```python
from build123d import *

# Parameters (mm, degrees)
F0_W     = 7.25
F0_H     = 3.25
F1_DEPTH = 3


with BuildPart() as f1:
    # F0 (on Top) → F1 (new body)
    with BuildSketch(Plane.XY):
        Polygon((9.582664, 28.182806), (4.046888, 28.182806), (-1.488889, 28.182806), (-11.920412, 38.29651), (-20.548956, 38.811646), (-21.450445, 36.493532), (-36.131848, 37.266236), (-36.775768, 39.455567), (-45.790665, 40.228274), (-51.328391, 34.561768), (-51.714741, 26.577145), (-47.207296, 25.546871), (-45.919452, 27.607419), (-31.366833, 24.001461), (-31.238047, 21.554559), (-26.953112, 20.524286), (-26.953112, 11.682806), (-26.953112, 2.841327), (-31.238047, 1.811053), (-31.366833, -0.635848), (-45.919452, -4.241806), (-47.207296, -2.181258), (-51.714741, -3.211532), (-51.328391, -11.196155), (-45.790665, -16.862661), (-36.775768, -16.089954), (-36.131848, -13.900623), (-21.450445, -13.127919), (-20.548956, -15.446034), (-11.920412, -14.930897), (-1.488889, -4.817194), (4.046888, -4.817194), (9.582664, -4.817194), (20.014187, -14.930897), (28.642732, -15.446034), (29.54422, -13.127919), (44.225623, -13.900623), (44.869543, -16.089954), (53.88444, -16.862661), (59.422166, -11.196155), (59.808516, -3.211532), (55.301071, -2.181258), (54.013227, -4.241806), (39.460608, -0.635848), (39.331823, 1.811053), (35.046888, 2.841327), (35.046888, 20.524286), (39.331823, 21.554559), (39.460608, 24.001461), (54.013227, 27.607419), (55.301071, 25.546871), (59.808516, 26.577145), (59.422166, 34.561768), (53.88444, 40.228274), (44.869543, 39.455567), (44.225623, 37.266236), (29.54422, 36.493532), (28.642732, 38.811646), (20.014187, 38.29651), align=None)
        Polygon((-47.588665, -8.516893), (-28.300909, -4.230727), (-26.597083, -9.545867), (-39.028991, -10.319404), (-39.857782, -12.695283), (-44.388525, -12.86104), (-47.648445, -9.766877), align=None, mode=Mode.SUBTRACT)
        with Locations((-11.828112, -3.192194)):
            Rectangle(F0_W, F0_H, mode=Mode.SUBTRACT)
        with Locations((19.921888, -3.192194)):
            Rectangle(F0_W, F0_H, mode=Mode.SUBTRACT)
        Polygon((34.690858, -9.545867), (36.394685, -4.230727), (55.68244, -8.516893), (55.74222, -9.766877), (52.482301, -12.86104), (47.951558, -12.695283), (47.122766, -10.319404), align=None, mode=Mode.SUBTRACT)
        Polygon((-9.203112, 9.764191), (-9.203112, 11.682806), (-9.203112, 13.601422), (-5.139121, 14.579791), (-5.063862, 15.55816), (-3.483421, 16.31075), (-2.580312, 15.934454), (0.806347, 17.364377), (0.430051, 18.192228), (2.010493, 18.944819), (4.046888, 18.944819), (6.083283, 18.944819), (7.663724, 18.192228), (7.287428, 17.364377), (10.674088, 15.934454), (11.577197, 16.31075), (13.157638, 15.55816), (13.232897, 14.579791), (17.296888, 13.601422), (17.296888, 11.682806), (17.296888, 9.764191), (13.232897, 8.785822), (13.157638, 7.807453), (11.577197, 7.054863), (10.674088, 7.431159), (7.287428, 6.001236), (7.663724, 5.173385), (6.083283, 4.420794), (4.046888, 4.420794), (2.010493, 4.420794), (0.430051, 5.173385), (0.806347, 6.001236), (-2.580312, 7.431159), (-3.483421, 7.054863), (-5.063862, 7.807453), (-5.139121, 8.785822), align=None, mode=Mode.SUBTRACT)
        Polygon((-26.597083, 32.911479), (-28.300909, 27.59634), (-47.588665, 31.882506), (-47.648445, 33.13249), (-44.388525, 36.226653), (-39.857782, 36.060896), (-39.028991, 33.685017), align=None, mode=Mode.SUBTRACT)
        with Locations((-11.828112, 26.557806)):
            Rectangle(F0_W, F0_H, mode=Mode.SUBTRACT)
        with Locations((19.921888, 26.557806)):
            Rectangle(F0_W, F0_H, mode=Mode.SUBTRACT)
        Polygon((36.394685, 27.59634), (34.690858, 32.911479), (47.122766, 33.685017), (47.951558, 36.060896), (52.482301, 36.226653), (55.74222, 33.13249), (55.68244, 31.882506), align=None, mode=Mode.SUBTRACT)
    extrude(amount=F1_DEPTH)


solid = f1.part
```
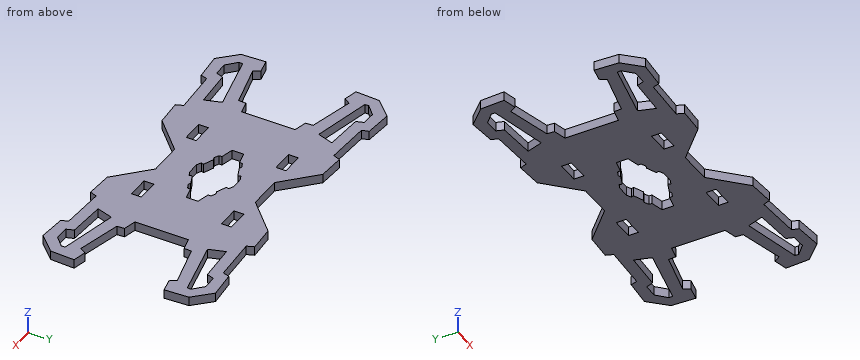
Here's how the part is built. I have some questions about the finished solid (model axes, mm). Coordinates: 2 decimals unless noted, no trailing zeros. Loops run counter-clockwise (first coordinate to the right, second up) from the corner with the lowest first, then second, coordinate; pieces in that order, holes last. Notation, with made-up numbers: M -2.5,-10.75 L 40.5,-10.75 A6 ccw 40.5,-2.75 Z; hole C -40,-20.5 d1. An arc over 180 degrees is marked long. One line per item, written item: value.
1. Imagine slicing it at A-A (y = 11.5). List the corners of the cut face in (x, z) for me, and give its area (4 significant figures).
Geometry says:
outline: M -26.95,0 L -9.2,0 L -9.2,3 L -26.95,3 Z; M 17.3,0 L 35.05,0 L 35.05,3 L 17.3,3 Z
area: 106.5 mm2
2. Will these pins go through, and if not, where does the flat tip stop? pin 1 Ø4 at (x, y) = (-27.5, 10) entering from +Z; pin 2 Ø1.5 at (y, z) = (5, 2.5) entering from -X.
Geometry says:
pin 1: stops at z = 3
pin 2: stops at x = -26.95
3. Please list where these lines run through material, in increasing order: probe 1 along Y at (x, z) = (20, 1.2); probe 2 along Y at (x, z) = (23, 1.05); probe 3 along X at (y, z) = (8.5, 1.95).
Geometry says:
probe 1: y = -14.92 to -4.82, -1.57 to 24.93, 28.18 to 38.28
probe 2: y = -15.11 to -4.82, -1.57 to 24.93, 28.18 to 38.47
probe 3: x = -26.95 to -5.12, 13.21 to 35.05
4. Imagine slicing it at C-C (z = 2.3). State how many separate pieces and enclosed holes the cut face has, and give its area (3 significant figures).
Geometry says:
separate pieces: 1
enclosed holes: 9
area: 3,420 mm2
5. Imagine slicing it at D-D (x = 31.5). List the corners of the cut face in (y, z) for me.
Geometry says:
outline: M -13.23,0 L 36.6,0 L 36.6,3 L -13.23,3 Z
6. Imagine slicing it at B-B (x = -33). List the corners of the cut face in (y, z) for me.
Geometry says:
outline: M -13.74,0 L -9.94,0 L -9.94,3 L -13.74,3 Z; M -5.27,0 L -1.04,0 L -1.04,3 L -5.27,3 Z; M 24.41,0 L 28.64,0 L 28.64,3 L 24.41,3 Z; M 33.31,0 L 37.1,0 L 37.1,3 L 33.31,3 Z
